from build123d import *

# Parameters (mm, degrees)
F1_DEPTH = 51.5
F2_W     = 13
F2_H     = 22.75
F3_DEPTH = 13
F4_W     = 13
F4_H     = 3
F5_DEPTH = 5


with BuildPart() as f1:
    # F0 (on Front) → F1 (new body)
    with BuildSketch(Plane.XZ):
        Polygon((-10.25, 26.803684), (-29.5, 0), (-5, 0), (-5, 8.67), (5, 8.67), (5, 0), (29.5, 0), (10.25, 26.803684), align=None)
    extrude(amount=F1_DEPTH)

    # F2 (on face) → F3 (cut)
    with BuildSketch(Plane.XZ.offset(51.5)):
        with Locations((0, 15.428684)):
            Rectangle(F2_W, F2_H)
    extrude(amount=-F3_DEPTH, mode=Mode.SUBTRACT)

    # F4 (on face) → F5 (cut)
    with BuildSketch(Plane.XZ.offset(38.5)):
        with Locations((0, 23.303684)):
            Rectangle(F4_W, F4_H)
    extrude(amount=-F5_DEPTH, mode=Mode.SUBTRACT)


solid = f1.part
Geometry check sheet. Reference: the model listing, model coordinates, mm. A direction names the side the tool comes from. Give positions to 0.01 mm unless a question says otherwise; leave off trailing zeros. Write each loop counter-clockwise with the first axis right and the second up, starting at its lowest first coordinate (ties: lowest second). Pieces come first, ordered by that corner, then holes. Notation, with made-up numbers: (8, 9) - (44, 9) arc R24 ccw to (44, 29) - close; hole circle Ø2 at (85.25, -34). An arc over 180 degrees is marked (long way). Put each result on its own line as item: value.
1. Sectioned sample at B-B, the plane z = 4.75. Enter the section's corners in (x, y).
Ans:
outline: (-26.09, -51.5) - (-6.5, -51.5) - (-6.5, -38.5) - (-5, -38.5) - (-5, 0) - (-26.09, 0) - close; (5, -38.5) - (6.5, -38.5) - (6.5, -51.5) - (26.09, -51.5) - (26.09, 0) - (5, 0) - close
2. Sectioned sample at C-C, the plane x = -2. Enter the section's corners in (y, z).
Ans:
outline: (-38.5, 8.67) - (0, 8.67) - (0, 26.8) - (-38.5, 26.8) - (-38.5, 24.8) - (-33.5, 24.8) - (-33.5, 21.8) - (-38.5, 21.8) - close
3. Thickness scan on line 1 (X direction, y = -45.5, z = 1.5); line 2 (X direction, y = -20, z = 6); line 3 (Z direction, x = 0.5, y = -10). Record the ranges inside material, lowest first.
Ans:
line 1: x = -28.42 to -5, 5 to 28.42
line 2: x = -25.19 to -5, 5 to 25.19
line 3: z = 8.67 to 26.8
4. Go/stop test with flat-tipped pins: pin 1 (3.5 mm diameter, centred on x = -2, z = 22.5, fed in from -Y); pin 2 (1.5 mm diameter, centred on y = -45, z = 3.5, fed in from -X) (3 decimals); pin 3 (2.5 mm diameter, centred on y = -20.5, z = 4.5, fed in from -X). Record where each tip stops, or that it passes through.
Ans:
pin 1: stops at y = -38.5
pin 2: stops at x = -27.525
pin 3: stops at x = -27.17
5. Set-up check for faces 4 (the flat face through (6, -45, 4.054)), 5 (the flat face through (5, -25, 4)), 6 (the flat face through (0, -33.5, 23)): record each of +Z, -Z, +X, -X, +Y, -Y from which the full face is reachable in a straight line by a thin tool's end or side.
Ans:
face 4: +Z, -Y
face 5: -Z, +Y, -Y
face 6: -Y
6. Sectioned sample at A-A, the plane y = -46. Enter the section's corners in (x, z), plus the area to 3 significant figures.
Ans:
outline: (-29.5, 0) - (-5, 0) - (-5, 4.05) - (-6.5, 4.05) - (-6.5, 26.8) - (-10.25, 26.8) - close; (5, 0) - (29.5, 0) - (10.25, 26.8) - (6.5, 26.8) - (6.5, 4.05) - (5, 4.05) - close
area: 729 mm²
7. Draft check along X on faces 1 (the flat face through (0, 0, 11)), 2 (the flat face through (20.01, -25.39, 13.214)), 3 (the flat face through (0, -36, 21.804)). Enter one of: +X half, -X half, draft (parallel to the pull), parting line (faces both ways), or undercut.
Ans:
face 1: draft
face 2: +X half
face 3: undercut
8. Sectioned sample at D-D, the plane y = -16. Enter the section's corners in (x, z).
Ans:
outline: (-29.5, 0) - (-5, 0) - (-5, 8.67) - (5, 8.67) - (5, 0) - (29.5, 0) - (10.25, 26.8) - (-10.25, 26.8) - close
